```python
from build123d import *

# Parameters (mm, degrees)
SKETCH1_W           = 49.784
SKETCH1_H           = 23.876
BOSS_EXTRUDE1_DEPTH = 25.4
SHELL1_T            = -2.54
CUT_EXTRUDE1_REACH  = 44.835
SKETCH2_R           = 8.255
CUT_EXTRUDE2_REACH  = 37.843
SKETCH4_W           = 11.684
SKETCH4_H           = 17.78
SKETCH5_R           = 10.541
SKETCH5_R_2         = 8.128
BOSS_EXTRUDE3_DEPTH = 1.27
BOSS_EXTRUDE4_DEPTH = 12.7
SKETCH8_W           = 6.35
SKETCH8_H           = 5.08
BOSS_EXTRUDE5_DEPTH = 6.35
SKETCH9_W           = 22.86
SKETCH9_H           = 18.796
CUT_EXTRUDE3_DEPTH  = 1.524
SKETCH10_W          = 22.86
SKETCH10_H          = 18.796
CUT_EXTRUDE4_DEPTH  = 1.524
CHAMFER1_SIZE       = 1.27
SKETCH11_W          = 49.784
SKETCH11_H          = 25.4
CUT_EXTRUDE5_DEPTH  = 1.524


with BuildPart() as part:
    # Sketch1 → Boss-Extrude1 (new body)
    with BuildSketch(Plane.XY):
        Rectangle(SKETCH1_W, SKETCH1_H)
    extrude(amount=-BOSS_EXTRUDE1_DEPTH)

    # Shell1
    shell1_openings = [part.faces().sort_by_distance(p)[0] for p in [
        (0, 0, 0),
    ]]
    offset(amount=SHELL1_T, openings=shell1_openings, kind=Kind.INTERSECTION)

    # Sketch2 → Cut-Extrude1 (cut, up to next)
    with BuildSketch(Plane.XZ.offset(11.938), mode=Mode.PRIVATE) as cut_extrude1_sk1:
        with Locations(Location((-12.7, -11.684, 0), (0, 0, 270))):
            Circle(SKETCH2_R)
    cut_extrude1_tool1 = extrude(cut_extrude1_sk1.sketch, amount=-CUT_EXTRUDE1_REACH, mode=Mode.PRIVATE) & part.part
    # Sketch2 → Cut-Extrude1 (cut, up to next)
    with BuildSketch(Plane.XZ.offset(11.938), mode=Mode.PRIVATE) as cut_extrude1_sk2:
        with Locations(Location((12.7, -11.684, 0), (0, 0, 270))):
            Circle(SKETCH2_R)
    cut_extrude1_tool2 = extrude(cut_extrude1_sk2.sketch, amount=-CUT_EXTRUDE1_REACH, mode=Mode.PRIVATE) & part.part
    add(cut_extrude1_tool1.solids().sort_by_distance((-12.7, -11.938, -11.684))[0], mode=Mode.SUBTRACT)
    add(cut_extrude1_tool2.solids().sort_by_distance((12.7, -11.938, -11.684))[0], mode=Mode.SUBTRACT)

    # Sketch4 → Cut-Extrude2 (cut, up to next)
    with BuildSketch(Plane.XY.offset(-22.86), mode=Mode.PRIVATE) as cut_extrude2_sk1:
        with Locations((0, 0.508)):
            Rectangle(SKETCH4_W, SKETCH4_H)
    cut_extrude2_tool1 = extrude(cut_extrude2_sk1.sketch, amount=-CUT_EXTRUDE2_REACH, mode=Mode.PRIVATE) & part.part
    add(cut_extrude2_tool1.solids().sort_by_distance((0, 0.508, -22.86))[0], mode=Mode.SUBTRACT)

    # Sketch5 → Boss-Extrude3 (add)
    # profile 1 of 2: a face of its own
    with BuildSketch(Plane.XZ.offset(11.938)):
        with Locations(Location((-12.7, -11.684, 0), (0, 0, 270))):
            Circle(SKETCH5_R)
        with Locations(Location((-12.7, -11.684, 0), (0, 0, 270))):
            Circle(SKETCH5_R_2, mode=Mode.SUBTRACT)
    # profile 2 of 2: a face of its own
    with BuildSketch(Plane.XZ.offset(11.938)):
        with Locations(Location((12.7, -11.684, 0), (0, 0, 270))):
            Circle(SKETCH5_R)
        with Locations(Location((12.7, -11.684, 0), (0, 0, 270))):
            Circle(SKETCH5_R_2, mode=Mode.SUBTRACT)
    extrude(amount=BOSS_EXTRUDE3_DEPTH)

    # Sketch7 → Boss-Extrude4 (add)
    with BuildSketch(Plane(origin=(0, 0, -25.4), x_dir=(-1, 0, 0), z_dir=(0, 0, -1))):
        Polygon((-24.892, 2.522876328), (-24.892, -2.557123672), (-12.192, -2.557123672), (-12.192, 2.516226298), align=None)
    extrude(amount=BOSS_EXTRUDE4_DEPTH)

    # Sketch8 → Boss-Extrude5 (add)
    with BuildSketch(Plane(origin=(24.892, 0, 0), x_dir=(0, 0, -1), z_dir=(1, 0, 0))):
        with Locations((34.925, -0.017123672)):
            Rectangle(SKETCH8_W, SKETCH8_H)
    extrude(amount=BOSS_EXTRUDE5_DEPTH)

    # Sketch9 → Cut-Extrude3 (cut)
    with BuildSketch(Plane(origin=(-22.352, 0, 0), x_dir=(0, 0, -1), z_dir=(1, 0, 0))):
        with Locations((11.43, 0)):
            Rectangle(SKETCH9_W, SKETCH9_H)
    extrude(amount=-CUT_EXTRUDE3_DEPTH, mode=Mode.SUBTRACT)

    # Sketch10 → Cut-Extrude4 (cut)
    with BuildSketch(Plane.ZY.offset(-22.352)):
        with Locations((-11.43, 0)):
            Rectangle(SKETCH10_W, SKETCH10_H)
    extrude(amount=-CUT_EXTRUDE4_DEPTH, mode=Mode.SUBTRACT)

    # Chamfer1
    chamfer1_edges = [part.edges().sort_by_distance(p)[0] for p in [
        (-12.7, -13.208, -1.143),
        (12.7, -13.208, -1.143),
    ]]
    chamfer(chamfer1_edges, length=CHAMFER1_SIZE - 0.0001)  # a hair under: the kernel refuses the full size

    # Sketch11 → Cut-Extrude5 (cut)
    with BuildSketch(Plane(origin=(0, 11.938, 0), x_dir=(1, 0, 0), z_dir=(0, 1, 0))):
        with Locations((0, 12.7)):
            Rectangle(SKETCH11_W, SKETCH11_H)
    extrude(amount=-CUT_EXTRUDE5_DEPTH, mode=Mode.SUBTRACT)


solid = part.part
```
Here's how the part is built. I have some questions about the finished solid (model axes, mm). A direction names the side the tool comes from. Round coordinates to 2 decimals unless told otherwise and drop trailing zeros. Loops run counter-clockwise (first coordinate to the right, second up) from the corner with the lowest first, then second, coordinate; pieces in that order, holes last.
1. Will these pins go through, and if not, where does the flat tip stop? pin 1 (10 mm diameter, centred on x = -3.5, z = -19.5, fed in from -Y); pin 2 (4 mm diameter, centred on x = 29, y = 0.5, fed in from +Z); pin 3 (5 mm diameter, centred on x = -18.5, y = -4.5, fed in from +Z); pin 4 (14.5 mm diameter, centred on x = 12.7, z = -11.684, fed in from -Y).
Answers:
pin 1: stops at y = -13.21
pin 2: stops at z = -31.75
pin 3: stops at z = -22.86
pin 4: stops at y = 9.4
2. For faces 1 (the face through (28, 0, -31.75)), 2 (the face through (19, -2.557, -32)), 3 (the face through (-5.842, 0, -24)), 4 (the face through (23.876, 0, -12)), 5 (the face through (12.192, 0, -32)), which set-ups out of +Z, -Z, +X, -X, +Y, -Y let a thin tool reach every point of the face, with its end or its side?
Answers:
face 1: +Z, +X, +Y, -Y
face 2: -Z, +X, -X, -Y
face 3: +Z, -Z
face 4: +Z
face 5: -Z, -X, +Y, -Y
3. Suppose I cut it at A-A, the plane y = -1. Please give me the cut outline in (x, z).
Answers:
outline: (-24.89, -25.4) - (-5.84, -25.4) - (-5.84, -22.86) - (-23.88, -22.86) - (-23.88, 0) - (-24.89, 0) - close; (5.84, -25.4) - (12.19, -25.4) - (12.19, -38.1) - (31.24, -38.1) - (31.24, -31.75) - (24.89, -31.75) - (24.89, 0) - (23.88, 0) - (23.88, -22.86) - (5.84, -22.86) - close
4. If I drill on probe 1 along X at (y, z) = (0.5, -7); probe 2 along Y at (x, z) = (-4, -9.5); probe 3 along Y at (x, z) = (14, -11.5), over which ranges is the centre line in solid material (lowest first)?
Answers:
probe 1: x = -24.89 to -23.88, 23.88 to 24.89
probe 2: y = -13.21 to -9.4, 9.4 to 10.41
probe 3: y = 9.4 to 10.41
5. Suppose I cut it at C-C, the plane y = -11.25. Please give me the cut outline in (x, z) (3 decimals), and give its area (3 significant figures).
Answers:
outline: (-24.892, -25.4) - (24.892, -25.4) - (24.892, 0) - (-24.892, 0) - close; hole circle Ø16.51 at (-12.7, -11.684); hole circle Ø16.51 at (12.7, -11.684)
area: 836 mm2
6. Thinking about a two-plate mould opening in Z: for faces 6 (the face through (15.141, -12.564, -19.437)), 7 (the face through (0, 9.398, -13)), 8 (the face through (-6, -10, 0)), which applies, released by +Z, released by -Z, zero draft, split by the parting line, or undercut?
Answers:
face 6: undercut
face 7: zero draft
face 8: released by +Z
